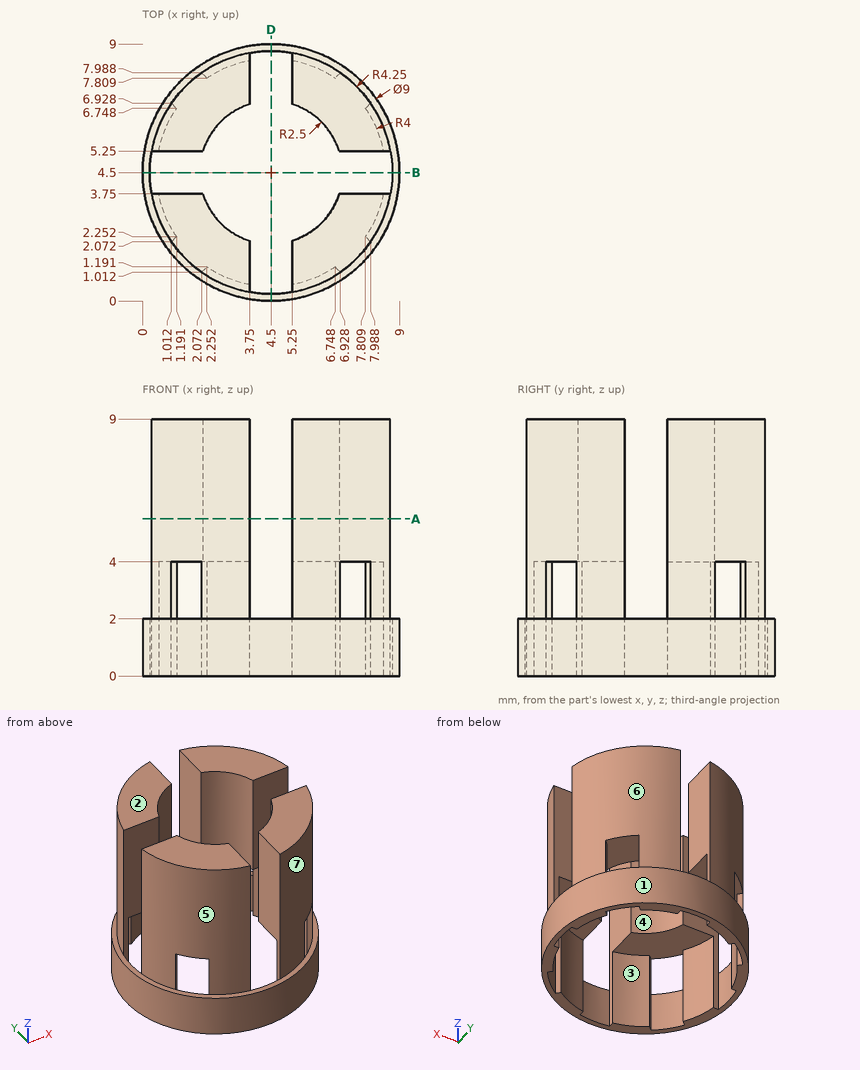
Could you check a few things on this drawing? It's one solid part, dimensions in mm from its lowest x, y, z. A direction names the side the tool comes from. Round coordinates to 2 decimals unless told otherwise and drop trailing zeros. Loops run counter-clockwise (first coordinate to the right, second up) from the corner with the lowest first, then second, coordinate; pieces in that order, holes last.
Q1. I want a section at B-B (y = 4.5). Write out the boundary of the cut face in (x, z).
Q2. On a 3-axis mill with a long thin cutter (end or side, diameter ignored), from which of +Z, -Z, +X, -X, +Y, -Y can I reach the whole of each face in a straight line? I mean the marked faces 5, 6 and 7. Say none if no direction works.
Q3. Thinking about a two-plate mould opening in X: for the marked faces 1, 2, 3 and 4, which applies, pulls with the +X half, pulls with the -X half, needs draft (parallel to the pull), parting line crosses it, or undercut?
Q4. I want a section at A-A (z = 5.5). Give the number of separate pieces and of enclosed holes in the cut face.
Q5. For P1, Ø0.5, axis at x = 1, z = 5.5, coming from the -Y side; P2, Ø4, axis at y = 5, z = 8, coming from the -X side; P3, Ø0.5, axis at y = 1.5, z = 3, coming from the -X side; P4, Ø0.5, axis at x = 1.5, z = 4, coming from the +Y side, each with a flat end and sliding along its axis, tell me the tip position at first contact or that it passes through.
Q6. Please list where these lines run through material, in increasing order: L1, parallel to Z at x = 2, y = 6.5; L2, parallel to Y at x = 8, z = 6.5; L3, parallel to Y at x = 1.25, z = 6.5.
Answer below:
1. outline: (0, 0) - (0.25, 0) - (0.25, 2) - (0, 2) - close; (8.75, 0) - (9, 0) - (9, 2) - (8.75, 2) - close
2. face 5: +Z, -X, -Y
2. face 6: +Z, +X, +Y
2. face 7: +Z, +X, -Y
3. face 1: parting line crosses it
3. face 2: needs draft
3. face 3: undercut
3. face 4: undercut
4. separate pieces: 4
4. enclosed holes: 0
5. P1: stops at y = 1.76
5. P2: stops at x = 0.32
5. P3: passes through
5. P4: stops at y = 7.74
6. L1: z = 4 to 9
6. L2: y = 2.09 to 3.75, 5.25 to 6.91
6. L3: y = 1.76 to 3.75, 5.25 to 7.24
